from build123d import *

# Parameters (mm, degrees)
CROQUIS1_R              = 1.5
SALIENTE_EXTRUIR1_DEPTH = 3
CROQUIS3_W              = 22
CROQUIS3_H              = 37
SALIENTE_EXTRUIR2_DEPTH = 13
CORTAR_EXTRUIR1_START   = -37
CORTAR_EXTRUIR1_DEPTH   = 37
SALIENTE_EXTRUIR4_DEPTH = 6
CROQUIS7_W              = 3.002058729
CROQUIS7_H              = 21
CORTAR_EXTRUIR2_DEPTH   = 22
CROQUIS8_W              = 3
CROQUIS8_H              = 43
SALIENTE_EXTRUIR5_DEPTH = 25
SALIENTE_EXTRUIR6_START = -19
SALIENTE_EXTRUIR6_DEPTH = 19
CROQUIS13_W             = 1
CROQUIS13_H             = 2
CROQUIS13_H_2           = 5
SALIENTE_EXTRUIR8_DEPTH = 1.5


with BuildPart() as part:
    # Croquis1 → Saliente-Extruir1 (new body)
    with BuildSketch(Plane.XY):
        with BuildLine():
            Line((-56.197309417, 29.461883408), (-56.197309417, 24.961883408))
            Line((-56.197309417, 24.961883408), (-49.197309417, 17.961883408))
            Line((-49.197309417, 17.961883408), (-49.197309417, 4.961883408))
            Line((-49.197309417, 4.961883408), (-56.197309417, 4.961883408))
            Line((-56.197309417, 4.961883408), (-56.197309417, 0.461883408))
            ThreePointArc((-56.197309417, 0.461883408), (-55.099110766, -2.293519818), (-52.406664651, -3.538116592))
            Line((-52.406664651, -3.538116592), (-4.197309417, -3.538116592))
            Line((-4.197309417, -3.538116592), (-4.197309417, 7.961883408))
            Line((-4.197309417, 7.961883408), (-10.197309417, 7.961883408))
            Line((-10.197309417, 7.961883408), (-10.197309417, 15.961883408))
            Line((-10.197309417, 15.961883408), (-4.197309417, 21.961883408))
            Line((-4.197309417, 21.961883408), (-4.197309417, 33.461883408))
            Line((-4.197309417, 33.461883408), (-52.197309417, 33.461883408))
            ThreePointArc((-52.197309417, 33.461883408), (-55.025736542, 32.290310533), (-56.197309417, 29.461883408))
        make_face()
        with Locations((-52.19152813, 0.461883408)):
            Circle(CROQUIS1_R, mode=Mode.SUBTRACT)
        with Locations((-7.69152813, 0.461883408)):
            Circle(CROQUIS1_R, mode=Mode.SUBTRACT)
        with Locations((-52.197309417, 29.461883408)):
            Circle(CROQUIS1_R, mode=Mode.SUBTRACT)
        with Locations((-7.697309417, 29.461882832)):
            Circle(CROQUIS1_R, mode=Mode.SUBTRACT)
    extrude(amount=SALIENTE_EXTRUIR1_DEPTH)

    # Croquis3 → Saliente-Extruir2 (add)
    with BuildSketch(Plane.XY.offset(3)):
        with Locations((-38.197309417, 14.961883408)):
            Rectangle(CROQUIS3_W, CROQUIS3_H)
    extrude(amount=SALIENTE_EXTRUIR2_DEPTH)

    # Croquis4 → Cortar-Extruir1 (cut)
    with BuildSketch(Plane.XZ.offset(3.538116592).offset(CORTAR_EXTRUIR1_START)):
        Polygon((-27.197309417, 16), (-27.197309417, 6.002058729), (-49.197309417, 16), align=None)
    extrude(amount=CORTAR_EXTRUIR1_DEPTH, mode=Mode.SUBTRACT)

    # Croquis6 → Saliente-Extruir4 (add)
    with BuildSketch(Plane(origin=(0, 33.461883408, 0), x_dir=(1, 0, 0), z_dir=(0, 1, 0))):
        Polygon((-27.197309417, -6.002058729), (-49.197309417, -16), (-49.197309417, 0), (-27.197309417, 0), align=None)
    extrude(amount=SALIENTE_EXTRUIR4_DEPTH)

    # Croquis7 → Cortar-Extruir2 (cut)
    with BuildSketch(Plane(origin=(-27.197309417, 0, 0), x_dir=(0, 0, -1), z_dir=(1, 0, 0))):
        with Locations((-4.501029365, 25.961883408)):
            Rectangle(CROQUIS7_W, CROQUIS7_H)
    extrude(amount=-CORTAR_EXTRUIR2_DEPTH, mode=Mode.SUBTRACT)

    # Croquis8 → Saliente-Extruir5 (add)
    with BuildSketch(Plane(origin=(-2.394740987, 0, -5.269515022), x_dir=(0.9103985682863143, 0, -0.4137323372208525), z_dir=(0.4137323372208525, 0, 0.9103985682863143))):
        with Locations((-28.743637341, 17.961883408)):
            Rectangle(CROQUIS8_W, CROQUIS8_H)
    extrude(amount=SALIENTE_EXTRUIR5_DEPTH)

    # Croquis9 → Saliente-Extruir6 (add)
    with BuildSketch(Plane.XZ.offset(3.538116592).offset(SALIENTE_EXTRUIR6_START)):
        Polygon((-16.854000987, 28.762022936), (-27.197309417, 6.002058729), (-27.197309417, 3), (-16.854000987, 3), align=None)
    extrude(amount=SALIENTE_EXTRUIR6_DEPTH)

    # Croquis13 → Saliente-Extruir8 (add)
    with BuildSketch(Plane.XY.offset(3)):
        with Locations((-10.197309417, -2.538116592)):
            Rectangle(CROQUIS13_W, CROQUIS13_H)
        with Locations((-10.197309417, 32.461883408)):
            Rectangle(CROQUIS13_W, CROQUIS13_H)
        with Locations((-14.197309417, 30.961883408)):
            Rectangle(CROQUIS13_W, CROQUIS13_H_2)
        with Locations((-14.197309417, -1.038116592)):
            Rectangle(CROQUIS13_W, CROQUIS13_H_2)
    extrude(amount=SALIENTE_EXTRUIR8_DEPTH)


solid = part.part
Read the model definition and answer for the solid it produces. Units are mm, in the model's axes. A direction names the side the tool comes from. Coordinates: 2 decimals unless noted, no trailing zeros. Loops run counter-clockwise (first coordinate to the right, second up) from the corner with the lowest first, then second, coordinate; pieces in that order, holes last.
Q1. The part is cut by section B-B on z = 8. Write down the section's boundary in (x, y), and give its area (3 significant figures).
Q2. The part is cut by section C-C on y = 4. Write down the section's boundary in (x, z).
Q3. The mould has two halves that part along Y. Classify faces 5 (the face through (-28.6, -3.538, 8.5)), 6 (the face through (-9.697, -3, 4)), 7 (the face through (-25, 15.462, 9)), 8 (the face through (-10.197, 12, 1)): +Y half, -Y half, draft (parallel to the pull), parting line (faces both ways), or undercut.
Q4. Each of these flat-tipped pins is pushed along its axis until it touches: pin 1 Ø5 at (y, z) = (37.5, 2.5) entering from +X; pin 2 Ø1.5 at (x, y) = (-13.5, 27) entering from +Z; pin 3 Ø1.5 at (y, z) = (11.5, 2) entering from +X. Where does it stop, or does it pass through?
Q5. The part is cut by section A-A on y = 35.5. Write down the section's boundary in (x, z), and give its area (3 significant figures).
Q6. The part is cut by section D-D on x = -33. Write down the section's boundary in (y, z), and give its area (3 significant figures).
Q7. Consider probe 1 along Z at (x, y) = (-47, 24); probe 2 along Z at (x, y) = (-52.5, 26); probe 3 along X at (y, z) = (37, 5.5). Determine where each line is inside the solid, lowest interval first.
Q8. Which of the six approach directions +Z, -Z, +X, -X, +Y, -Y give full straight-line access (tool end or side, diameter ignored) to faces 1 (the face through (-16, 33.462, 2)), 2 (the face through (-54, 2, 3)), 3 (the face through (-7, 7.962, 1)), 4 (the face through (-13.697, -1, 4))?
Results below:
1. outline: (-49.2, -3.54) - (-31.59, -3.54) - (-31.59, 39.46) - (-49.2, 39.46) - close; (-29.58, -3.54) - (-16.85, -3.54) - (-16.85, 15.46) - (-26.29, 15.46) - (-26.29, 39.46) - (-29.58, 39.46) - close
1. area: 1,080 mm2
2. outline: (-56.2, 0) - (-4.2, 0) - (-4.2, 3) - (-16.85, 3) - (-16.85, 28.76) - (-19.59, 30) - (-29.93, 7.24) - (-49.2, 16) - (-49.2, 3) - (-56.2, 3) - close
3. face 5: -Y half
3. face 6: draft
3. face 7: undercut
3. face 8: undercut
4. pin 1: stops at x = -27.2
4. pin 2: stops at z = 3
4. pin 3: stops at x = -10.2
5. outline: (-49.2, 0) - (-27.2, 0) - (-27.2, 3) - (-49.2, 3) - close; (-49.2, 6) - (-27.2, 6) - (-16.85, 28.76) - (-19.59, 30) - (-29.93, 7.24) - (-49.2, 16) - close
5. area: 251 mm2
6. outline: (-3.54, 0) - (39.46, 0) - (39.46, 8.64) - (-3.54, 8.64) - close; hole (15.46, 3) - (36.46, 3) - (36.46, 6) - (15.46, 6) - close
6. area: 308 mm2
7. probe 1: z = 0 to 3, 6 to 15
7. probe 2: z = 0 to 3
7. probe 3: x = -49.2 to -27.2
8. face 1: -Z, +X, +Y
8. face 2: +Z, -X, +Y, -Y
8. face 3: +Z, -Z, +X
8. face 4: +Z, +Y, -Y
